Autodesk Inventor part; units mm, degrees
ref_plane "YZ Plane" through (0, 0, 0) normal (1, 0, 0) x (0, 1, 0)
ref_plane "XZ Plane" through (0, 0, 0) normal (0, 1, 0) x (-1, 0, 0)
ref_plane "XY Plane" through (0, 0, 0) normal (0, 0, 1) x (1, 0, 0)
sketch "Sketch1" plane through (0, 0, 0) normal (0, 0, 1) x (1, 0, 0)
  circle A0 centre (0, 0) radius 12.5
  dimension "d0" = 25
extrude "Extrusion1" add sketch "Sketch1" along normal blind 26.5
fillet "Fillet1" radius 1 2 edges at (-12.5, 0, 26.5) (-12.5, 0, 0)
sketch "Sketch2" plane through (0, 0, 26.5) normal (0, 0, 1) x (1, 0, 0)
  circle A0 centre (-5.9291, 5.7365) radius 1.75
  line L0 (-5.9291, 5.7365) -> (0, 0) construction
  line L1 (0, 0) -> (5.9291, -5.7365) construction
  circle A1 centre (5.9291, -5.7365) radius 1.75
  dimension "d5" = 3.5
  dimension "d6" = 3.5
  dimension "d7" = 16.5
extrude "Extrusion2" cut sketch "Sketch2" against normal blind 10
sketch "Sketch3" plane through (0, 0, 0) normal (0, 0, -1) x (-1, 0, 0)
  circle A0 centre (0, 0) radius 12.45
  dimension "d10" = 24.9
extrude "Extrusion3" add sketch "Sketch3" along normal blind 40
sketch "Sketch4" plane through (0, 0, 26.5) normal (0, 0, 1) x (1, 0, 0)
  circle A0 centre (0, 0) radius 2.5
  dimension "d13" = 5
extrude "Extrusion4" add sketch "Sketch4" along normal blind 30
sketch "Sketch5" plane through (0, 0, 56.5) normal (0, 0, 1) x (1, 0, 0)
  circle A0 centre (0, 0) radius 2.5
  line L0 (-2.0152, 1.4796) -> (2.0152, 1.4796)
  arc A1 (2.0152, 1.4796) -> (-2.0152, 1.4796) centre (0, 0) ccw
extrude "Extrusion5" cut sketch "Sketch5" against normal blind 8 contours L0 A0 picked at (0.5388, 1.6221)
fillet "Fillet2" radius 1 1 edges at (12.45, 0, -40)
properties part number "platform_motor"
For this review, take the finished solid that the model builds, in its own axes (mm). A direction names the side the tool comes from. Round coordinates to 2 decimals unless told otherwise and drop trailing zeros. Order: outer loops, then holes, each group sorted by start corner. A loop starts at its lowest first (then second) coordinate and runs counter-clockwise, first axis right, second up. Notation, with made-up numbers: (63.25, 12.5) -> (118.25, 12.5) arc R20 ccw to (118.25, 43.5) -> close; hole circle Ø11 at (27.25, 74). An arc over 180 degrees is marked (long way). Put each result on its own line as item: value.
Q1. Insertion check: pin 1 Ø10 at (y, z) = (3, -24) entering from -X; pin 2 Ø0.8 at (x, y) = (0, 2) entering from +Z; pin 3 Ø4.5 at (x, y) = (5.93, -5.74) entering from +Z. Each pin has a flat end and moves straight along its axis. Give the tip position at first contact, or say it passes through.
Check result:
pin 1: x = -12.45
pin 2: z = 48.5
pin 3: z = 26.5
Q2. Machinability: for faces 1 (the flat face through (-6, 6, 16.5)), 2 (the flat face through (0, 1.48, 53)), which of the approach directions +Z, -Z, +X, -X, +Y, -Y give a long, thin tool a straight path to every point of the face, cutting with its end or side? Answer none if there is none.
Check result:
face 1: +Z
face 2: +Z, +X, -X, +Y
Q3. Add section A-A on x = 0. Write out the cut boundary in (y, z), plus the area to 3 significant figures.
Check result:
outline: (-12.5, 1) arc R1 ccw to (-11.5, 0) -> (-12.45, 0) -> (-12.45, -39) arc R1 ccw to (-11.45, -40) -> (11.45, -40) arc R1 ccw to (12.45, -39) -> (12.45, 0) -> (11.5, 0) arc R1 ccw to (12.5, 1) -> (12.5, 25.5) arc R1 ccw to (11.5, 26.5) -> (2.5, 26.5) -> (2.5, 48.5) -> (1.48, 48.5) -> (1.48, 56.5) -> (-2.5, 56.5) -> (-2.5, 26.5) -> (-11.5, 26.5) arc R1 ccw to (-12.5, 25.5) -> close
area: 1,800 mm2
Q4. For probe 1 along Z at (x, y) = (-9, 0.5); probe 2 along X at (y, z) = (-0.25, -17.5); probe 3 along Y at (x, z) = (4.75, -17), list the stretches that pass through material, from the lowest coordinate up. Write a range as [from, to].
Check result:
probe 1: [-40, 26.5]
probe 2: [-12.45, 12.45]
probe 3: [-11.51, 11.51]
Q5. Add section D-D on z = 10.5. Write out the cut boundary in (x, y).
Check result:
outline: circle Ø25 at (0, 0)
Q6. Add section C-C on z = 44. Write out the cut boundary in (x, y).
Check result:
outline: circle Ø5 at (0, 0)
Q7. Add section B-B on y = 0. Write out the cut boundary in (x, z), plus the area to 3 significant figures.
Check result:
outline: (-12.5, 1) arc R1 ccw to (-11.5, 0) -> (-12.45, 0) -> (-12.45, -39) arc R1 ccw to (-11.45, -40) -> (11.45, -40) arc R1 ccw to (12.45, -39) -> (12.45, 0) -> (11.5, 0) arc R1 ccw to (12.5, 1) -> (12.5, 25.5) arc R1 ccw to (11.5, 26.5) -> (2.5, 26.5) -> (2.5, 56.5) -> (-2.5, 56.5) -> (-2.5, 26.5) -> (-11.5, 26.5) arc R1 ccw to (-12.5, 25.5) -> close
area: 1,810 mm2
